Part model, mm, in its own coordinate system. Give positions to 0.01 mm unless a question says otherwise; leave off trailing zeros. Order: outer loops, then holes, each group sorted by start corner. A loop starts at its lowest first (then second) coordinate and runs counter-clockwise, first axis right, second up.
1. Slice it at A-A on x = -158.75. List the corners of the cut face in (y, z).
2. Probe line 1 (Y direction, x = 88.9, z = 5); line 2 (Y direction, x = -7, z = 5.25); line 3 (X direction, y = 38.5, z = 1.75). List the from-to ranges inside material, lowest first.
3. Mould opens along Y. For faces 1 (the flat face through (-3, -76.2, 3)), 2 (the flat face through (-3, 1, 0)), 3 (the cylindrical face through (69.844, 54.254, 3.131)) say: +Y half, -Y half, draft (parallel to the pull), parting line (faces both ways), or undercut.
4. Drop a flat-ended pin along its axis: pin 1 Ø6 at (x, y) = (-127, 38.1) entering from +Z. Give the stop position or say it passes through.
from build123d import *

# Parameters (mm, degrees)
SKETCH1_W               = 368.3
SKETCH1_H               = 152.4
BOSS_EXTRUDE1_DEPTH     = 6.35
F_4_CLEARANCE_HOLE1_D   = 3.2639
F_1_4_CLEARANCE_HOLE1_D = 6.7564
F_1_4_CLEARANCE_HOLE2_D = 6.7564
SKETCH10_R              = 6.35
CUT_EXTRUDE1_DEPTH      = 200.394044545
F_2_CLEARANCE_HOLE1_D   = 2.4384
F_10_CLEARANCE_HOLE2_D  = 5.1054
F_10_CLEARANCE_HOLE1_D  = 5.1054
F_10_CLEARANCE_HOLE3_D  = 5.1054


with BuildPart() as part:
    # Sketch1 → Boss-Extrude1 (new body)
    with BuildSketch(Plane.XY):
        Rectangle(SKETCH1_W, SKETCH1_H)
    extrude(amount=BOSS_EXTRUDE1_DEPTH)

    # #4 Clearance Hole1 (through all)
    with Locations(Plane(origin=(0, 0, 0), x_dir=(-1, 0, 0), z_dir=(0, 0, -1))):
        with Locations((-174.752, 19.05), (-82.55, -53.34), (-174.752, -53.34), (-82.55, 19.05)):
            Hole(F_4_CLEARANCE_HOLE1_D / 2)

    # 1/4 Clearance Hole1 (through all)
    with Locations(Plane(origin=(0, 0, 0), x_dir=(-1, 0, 0), z_dir=(0, 0, -1))):
        with Locations((-158.75, 66.675), (158.75, -66.675), (-158.75, -66.675), (158.75, 66.675)):
            Hole(F_1_4_CLEARANCE_HOLE1_D / 2)

    # 1/4 Clearance Hole2 (through all)
    with Locations(Plane(origin=(0, 0, 0), x_dir=(-1, 0, 0), z_dir=(0, 0, -1))):
        with Locations((-177.8, 66.675), (177.8, -38.1), (-177.8, -38.1), (177.8, 66.675)):
            Hole(F_1_4_CLEARANCE_HOLE2_D / 2)

    # Sketch10 → Cut-Extrude1 (cut, through all)
    with BuildSketch(Plane(origin=(0, 0, 0), x_dir=(-1, 0, 0), z_dir=(0, 0, -1))):
        with Locations((-63.5, 53.975)):
            Circle(SKETCH10_R)
    extrude(amount=-CUT_EXTRUDE1_DEPTH, mode=Mode.SUBTRACT)

    # #2 Clearance Hole1 (through all)
    with Locations(Plane(origin=(0, 0, 0), x_dir=(-1, 0, 0), z_dir=(0, 0, -1))):
        with Locations((-133.35, 69.85), (-146.05, 69.85), (-120.65, 69.85), (-107.95, 69.85), (-95.25, 69.85), (-82.55, 69.85)):
            Hole(F_2_CLEARANCE_HOLE1_D / 2)

    # #10 Clearance Hole2 (through all)
    with Locations(Plane(origin=(0, 0, 0), x_dir=(-1, 0, 0), z_dir=(0, 0, -1))):
        with Locations((-146.05, 41.275), (-146.05, 28.575), (-95.25, 41.275), (-95.25, 28.575)):
            Hole(F_10_CLEARANCE_HOLE2_D / 2)

    # #10 Clearance Hole1 (through all)
    with Locations(Plane(origin=(0, 0, 0), x_dir=(-1, 0, 0), z_dir=(0, 0, -1))):
        with Locations((7, 38.1), (127, -36.9), (7, -36.9), (127, 38.1)):
            Hole(F_10_CLEARANCE_HOLE1_D / 2)

    # #10 Clearance Hole3 (through all)
    with Locations(Plane(origin=(0, 0, 0), x_dir=(-1, 0, 0), z_dir=(0, 0, -1))):
        with Locations((-133.35, -57.15), (-88.9, -69.85), (-133.35, -69.85), (-88.9, -57.15)):
            Hole(F_10_CLEARANCE_HOLE3_D / 2)


solid = part.part
Data:
1. outline: (-76.2, 0) - (-70.05, 0) - (-70.05, 6.35) - (-76.2, 6.35) - close; (-63.3, 0) - (63.3, 0) - (63.3, 6.35) - (-63.3, 6.35) - close; (70.05, 0) - (76.2, 0) - (76.2, 6.35) - (70.05, 6.35) - close
2. line 1: y = -76.2 to -72.4, -67.3 to -59.7, -54.6 to 76.2
2. line 2: y = -76.2 to -39.45, -34.35 to 35.55, 40.65 to 76.2
2. line 3: x = -184.15 to -129.52, -124.48 to -9.52, -4.48 to 184.15
3. face 1: -Y half
3. face 2: draft
3. face 3: undercut
4. pin 1: stops at z = 6.35
